Read the model definition and answer for the solid it produces. Units are mm, in the model's axes. Face numbers are marked on the shaded views. Coordinates: 2 decimals unless noted, no trailing zeros. Order: outer loops, then holes, each group sorted by start corner. A loop starts at its lowest first (then second) coordinate and runs counter-clockwise, first axis right, second up. Notation, with made-up numbers: M 1,46 L 58,46 A17 ccw 58,54 Z; hole C -38.5,-2.75 d10. An arc over 180 degrees is marked long. Use a Markdown table: item, result. Add a question column.
1) Find section C-C on x = -4.5. Write down the section's boundary in (y, z).
2) Find section A-A on x = 0. Write down the section's boundary in (y, z), plus the area to 3 significant figures.
3) Each of these flat-tipped pins is pushed along its axis until it touches: pin 1 Ø1.5 at (x, y) = (-4, 0) entering from -Z; pin 2 Ø1 at (x, z) = (3.5, 10) entering from -Y; pin 3 Ø5 at (y, z) = (1, 41.5) entering from +X; pin 4 Ø1.5 at (x, z) = (3, 13.5) entering from -Y. Where does it stop, or does it pass through?
4) The mould has two halves that part along Z. Classify the marked faces 1, 2, 3 and 4: released by +Z, released by -Z, zero draft, split by the parting line, or undercut.
5) Find section D-D on x = 4. Write down the section's boundary in (y, z), plus the area to 3 significant figures.
6) Find the intervals of material crossed by probe 1 along X at (y, z) = (0, 49.2); probe 2 along Z at (x, y) = (-4, -2.5); probe 3 along Y at (x, z) = (0, 29), in increasing order. Write a range as [from, to].
7) Find section B-B on z = 18.5. Write down the section's boundary in (x, y).
from build123d import *

# Parameters (mm, degrees)
BOX001_W          = 1.51
BOX001_H          = 9.5
BOX001_DEPTH      = 49.5
CHAMFER001_SIZE   = 1.5
BOX_W             = 5
BOX_H             = 20
BOX_DEPTH         = 60
CYLINDER005_R     = 1.25
CYLINDER005_DEPTH = 55
CYLINDER004_R     = 1.25
CYLINDER004_DEPTH = 55
CYLINDER007_R     = 1
CYLINDER007_DEPTH = 8
CYLINDER006_R     = 1
CYLINDER006_DEPTH = 8
CYLINDER002_R     = 5.25
CYLINDER002_DEPTH = 47.5
CYLINDER003_R     = 5.25
CYLINDER003_DEPTH = 47.5
CYLINDER001_R     = 3.25
CYLINDER001_DEPTH = 50.5
CHAMFER_SIZE      = 1
CYLINDER_R        = 7.25
CYLINDER_DEPTH    = 49.5


with BuildPart() as chamfer001:
    # Box001 → Box001 (new body)
    with BuildSketch(Plane(origin=(-6.76, -4.75, 0), x_dir=(1, 0, 0), z_dir=(0, 0, 1))):
        with Locations((0.755, 4.75)):
            Rectangle(BOX001_W, BOX001_H)
    extrude(amount=BOX001_DEPTH)

    # Chamfer001
    chamfer001_edges = [chamfer001.edges().sort_by_distance(p)[0] for p in [
        (-6.76, -4.75, 24.75),
        (-6.76, 4.75, 24.75),
    ]]
    chamfer(chamfer001_edges, length=CHAMFER001_SIZE)


with BuildPart() as cube:
    # Box → Box (new body)
    with BuildSketch(Plane(origin=(-11, -10, -4), x_dir=(1, 0, 0), z_dir=(0, 0, 1))):
        with Locations((2.5, 10)):
            Rectangle(BOX_W, BOX_H)
    extrude(amount=BOX_DEPTH)


with BuildPart() as cylinder005:
    # Cylinder005 → Cylinder005 (new body)
    with BuildSketch(Plane(origin=(-4, 0, 0), x_dir=(1, 0, 0), z_dir=(0, 0, 1))):
        Circle(CYLINDER005_R)
    extrude(amount=CYLINDER005_DEPTH)


with BuildPart() as cylinder004:
    # Cylinder004 → Cylinder004 (new body)
    with BuildSketch(Plane(origin=(4, 0, 0), x_dir=(1, 0, 0), z_dir=(0, 0, 1))):
        Circle(CYLINDER004_R)
    extrude(amount=CYLINDER004_DEPTH)


with BuildPart() as cylinder007:
    # Cylinder007 → Cylinder007 (new body)
    with BuildSketch(Plane(origin=(-4, 0, -0.5), x_dir=(0, 0, -1), z_dir=(1, 0, 0))):
        Circle(CYLINDER007_R)
    extrude(amount=CYLINDER007_DEPTH)


with BuildPart() as fusion002:
    # Cylinder006 → Cylinder006 (new body)
    with BuildSketch(Plane(origin=(-4, 0, 51), x_dir=(0, 0, -1), z_dir=(1, 0, 0))):
        Circle(CYLINDER006_R)
    extrude(amount=CYLINDER006_DEPTH)

    # Fusion002: union Cylinder005, Cylinder004, Cylinder007
    add(cylinder005.part)
    add(cylinder004.part)
    add(cylinder007.part)


with BuildPart() as cylinder002:
    # Cylinder002 → Cylinder002 (new body)
    with BuildSketch(Plane.XY.offset(1)):
        Circle(CYLINDER002_R)
    extrude(amount=CYLINDER002_DEPTH)


with BuildPart() as fusion001:
    # Cylinder003 → Cylinder003 (new body)
    with BuildSketch(Plane(origin=(5, 0, 1), x_dir=(1, 0, 0), z_dir=(0, 0, 1))):
        Circle(CYLINDER003_R)
    extrude(amount=CYLINDER003_DEPTH)

    # Fusion001: union Cylinder002
    add(cylinder002.part)


with BuildPart() as chamfer_body:
    # Cylinder001 → Cylinder001 (new body)
    with BuildSketch(Plane.XY):
        Circle(CYLINDER001_R)
    extrude(amount=CYLINDER001_DEPTH)

    # Chamfer
    chamfer_edges = [chamfer_body.edges().sort_by_distance(p)[0] for p in [
        (-3.25, 0, 50.5),
        (-3.25, 0, 0),
    ]]
    chamfer(chamfer_edges, length=CHAMFER_SIZE)


with BuildPart() as fusion003:
    # Cylinder → Cylinder (new body)
    with BuildSketch(Plane.XY):
        Circle(CYLINDER_R)
    extrude(amount=CYLINDER_DEPTH)

    # Fusion: union Chamfer body
    add(chamfer_body.part)

    # Cut: cut Fusion001
    add(fusion001.part, mode=Mode.SUBTRACT)

    # Cut001: cut Fusion002
    add(fusion002.part, mode=Mode.SUBTRACT)

    # Cut002: cut Cube
    add(cube.part, mode=Mode.SUBTRACT)

    # Fusion003: union Chamfer001
    add(chamfer001.part)


solid = fusion003.part
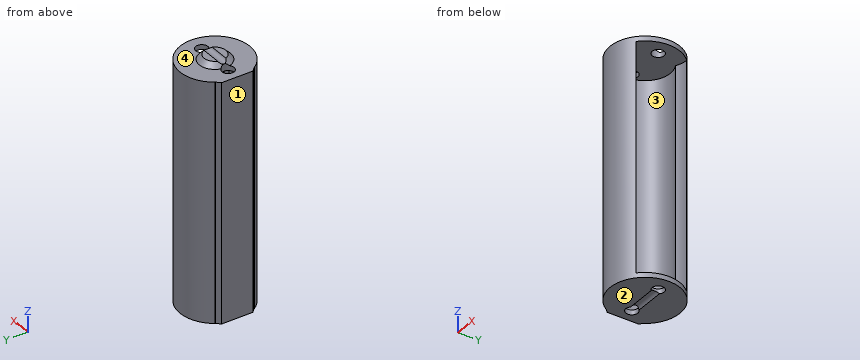
Check result:
| question | item | result |
|---|---|---|
| 1 | outline | M -5.68,0 L -1.15,0 L -1.15,1 L -2.7,1 L -2.7,48.5 L -1.15,48.5 L -1.15,49.5 L -5.68,49.5 Z; M 1.15,0 L 5.68,0 L 5.68,49.5 L 1.15,49.5 L 1.15,48.5 L 2.7,48.5 L 2.7,1 L 1.15,1 Z |
| 2 | outline | M -7.25,0 L -0.87,0 A1 cw 0.87,0 L 7.25,0 L 7.25,49.5 L 3.25,49.5 L 2.25,50.5 L 0.87,50.5 A1 cw -0.87,50.5 L -2.25,50.5 L -3.25,49.5 L -7.25,49.5 Z; hole M -5.25,1 L 5.25,1 L 5.25,48.5 L -5.25,48.5 Z |
| 2 | area | 223 mm2 |
| 3 | pin 1 | passes through |
| 3 | pin 2 | stops at y = -6.6 |
| 3 | pin 3 | stops at x = -3.91 |
| 3 | pin 4 | stops at y = -6.89 |
| 4 | face 1 | zero draft |
| 4 | face 2 | released by -Z |
| 4 | face 3 | undercut |
| 4 | face 4 | released by +Z |
| 5 | outline | M -6.05,0 L -1.25,0 L -1.25,1 L -5.15,1 L -5.15,48.5 L -1.25,48.5 L -1.25,49.5 L -6.05,49.5 Z; M 1.25,0 L 6.05,0 L 6.05,49.5 L 1.25,49.5 L 1.25,48.5 L 5.15,48.5 L 5.15,1 L 1.25,1 Z |
| 5 | area | 104 mm2 |
| 6 | probe 1 | x = [-6.76, -5.25], [-2.75, 2.75], [5.25, 7.25] |
| 6 | probe 2 | z = [0, 1], [48.5, 49.5] |
| 6 | probe 3 | y = [-7.25, -5.25], [5.25, 7.25] |
| 7 | outline | M -6.76,-3.25 L -6,-4.01 L -6,-4.07 A7.25 ccw 5,-5.25 A5.25 cw 2.5,-4.62 A5.25 cw long 2.5,4.62 A5.25 cw 5,5.25 A7.25 ccw -6,4.07 L -6,4.01 L -6.76,3.25 Z |
